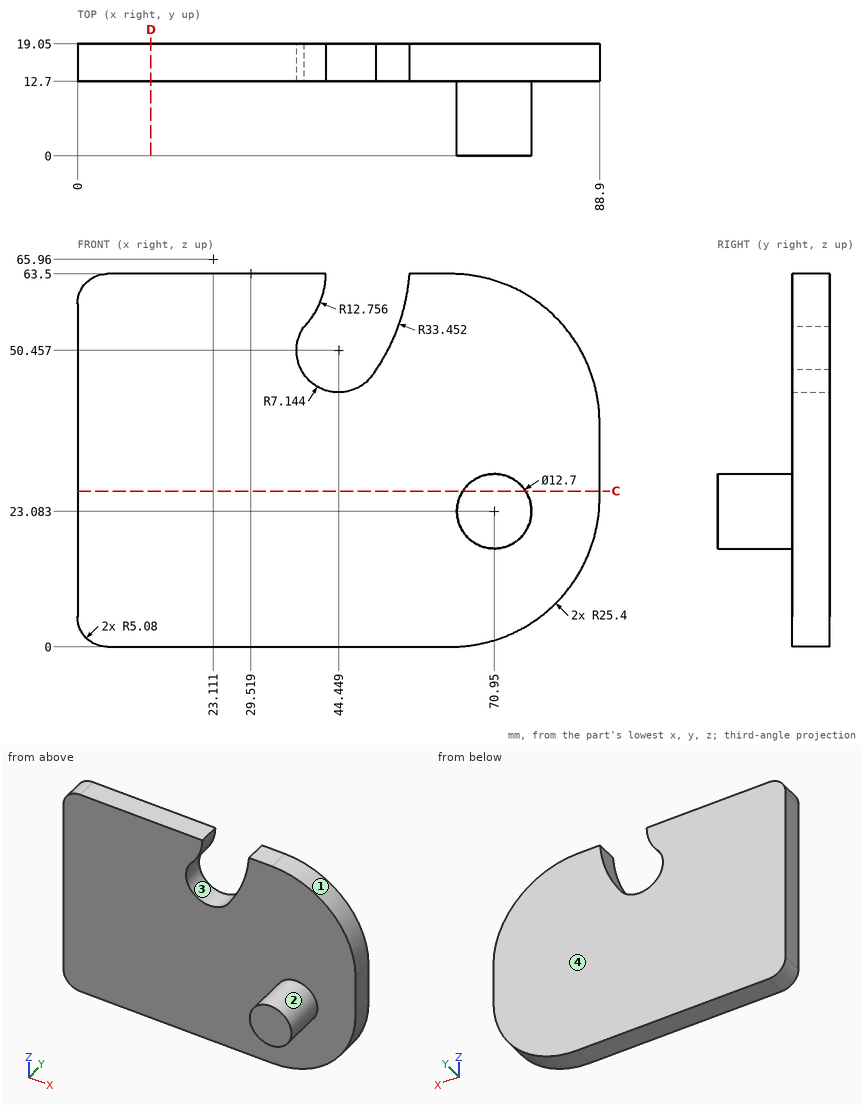
Design review of the part shown in the three views and the two pictorial views. Dimensions are in mm from the part's minimum x, y and z. Round coordinates to 2 decimals unless told otherwise and drop trailing zeros. Write each loop counter-clockwise with the first axis right and the second up, starting at its lowest first coordinate (ties: lowest second). Pieces come first, ordered by that corner, then holes. Notation, with made-up numbers: M 82,21.5 L 125,21.5 A23 cw 125,30.5 Z; hole C -39.5,57.25 d4. An arc over 180 degrees is marked long. One line per item, written item: value. Start each with the question number.
1. Draft analysis for pull direction Z (two halves, no side actions). For the marked faces 1, 2, 3 and 4, state which applies: pulls with the +Z half, pulls with the -Z half, needs draft (parallel to the pull), parting line crosses it, or undercut.
2. Take a section at D-D on x = 12.5. State the section outline as (y, z) points, then the cut area to 3 significant figures.
3. To check wall thickness, follow probe 1 along Y at (x, z) = (45, 24); probe 2 along Z at (x, y) = (38, 14) (1 decimal); probe 3 along X at (y, z) = (11, 18) (1 decimal). State the ranges of each line that lie inside material, in increasing order. Write a range as from..to.
4. Clearance check with flat-ended pins moving along their axes: P1, Ø3, axis at x = 63.5, z = 47, coming from the -Y side; P2, Ø1.5, axis at y = 16.5, z = 57, coming from the +X side; P3, Ø10, axis at y = 17, z = 47, coming from the +X side. State where each tip first meets the part, or that it passes through.
5. Take a section at C-C on z = 26.5. State the section outline as (x, y) points.
Computed:
1. face 1: pulls with the +Z half
1. face 2: parting line crosses it
1. face 3: undercut
1. face 4: needs draft
2. outline: M 12.7,0 L 19.05,0 L 19.05,63.5 L 12.7,63.5 Z
2. area: 403 mm²
3. probe 1: y = 12.7..19.05
3. probe 2: z = 0..47.4, 53.5..63.5
3. probe 3: x = 67.1..74.8
4. P1: stops at y = 12.7
4. P2: stops at x = 81.27
4. P3: stops at x = 88.6
5. outline: M 0,12.7 L 65.6,12.7 L 65.6,0 L 76.3,0 L 76.3,12.7 L 88.9,12.7 L 88.9,19.05 L 0,19.05 Z
